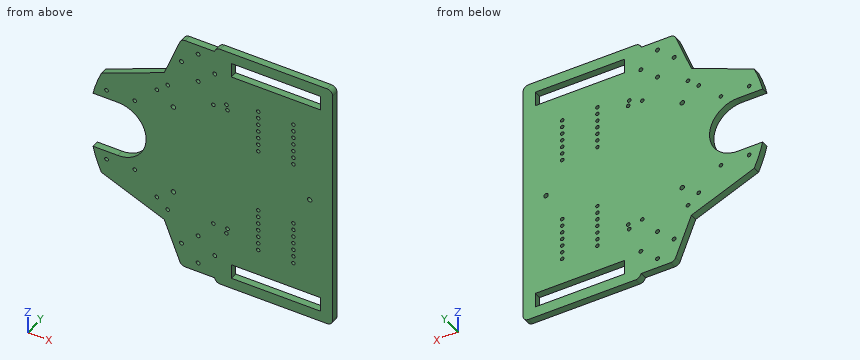
from build123d import *

# Parameters (mm, degrees)
BOSS_EXTRUDE1_DEPTH    = 6.35
SKETCH2_R              = 1.5875
SKETCH2_W              = 80.264
SKETCH2_H              = 12.954
CUT_EXTRUDE1_DEPTH     = 162.484606465
SKETCH7_R              = 2.032
CUT_EXTRUDE4_DEPTH     = 162.484606465
SKETCH8_R              = 1.651
CUT_EXTRUDE5_DEPTH     = 162.484606465
CUT_EXTRUDE6_DEPTH     = 160.416662013
SKETCH10_R             = 1.651
CUT_EXTRUDE7_DEPTH     = 160.416662013
SKETCH11_W             = 225
SKETCH11_H             = 6.35
BOSS_EXTRUDE2_DEPTH    = 8
FILLET2_R              = 5.08
SKETCH15_W             = 29.985408059
SKETCH15_H             = 4.069721463
CUT_EXTRUDE8_DEPTH     = 160.416662013
CUT_EXTRUDE9_START     = -6.35
CUT_EXTRUDE9_OUTLINE_R = 1.775
CUT_EXTRUDE9_DEPTH     = 6.35


# Read off the part's stored shape, not the designer's step: Cut-Extrude9
with BuildPart() as part:
    # Sketch1 → Boss-Extrude1 (new body)
    with BuildSketch(Plane(origin=(0, 0, 0), x_dir=(1, 0, 0), z_dir=(0, 1, 0))):
        with BuildLine():
            Line((-3.175, 112.5), (95.25, 112.5))
            Line((95.25, 112.5), (95.25, -112.5))
            Line((95.25, -112.5), (-3.175, -112.5))
            ThreePointArc((-3.175, -112.5), (-115.675, 0), (-3.175, 112.5))
        make_face()
    extrude(amount=-BOSS_EXTRUDE1_DEPTH)

    # Sketch2 → Cut-Extrude1 (cut, through all)
    with BuildSketch(Plane(origin=(0, 0, 0), x_dir=(1, 0, 0), z_dir=(0, 1, 0))):
        with Locations(Location((36.144045702, -66.3448, 0), (0, 0, 270))):
            Circle(SKETCH2_R)
        with Locations(Location((36.144045702, -59.9948, 0), (0, 0, 270))):
            Circle(SKETCH2_R)
        with Locations(Location((36.144045702, -53.6448, 0), (0, 0, 270))):
            Circle(SKETCH2_R)
        with Locations(Location((36.144045702, -47.2948, 0), (0, 0, 270))):
            Circle(SKETCH2_R)
        with Locations(Location((36.144045702, -40.9448, 0), (0, 0, 270))):
            Circle(SKETCH2_R)
        with Locations(Location((36.144045702, -34.5948, 0), (0, 0, 270))):
            Circle(SKETCH2_R)
        with Locations(Location((36.144045702, -28.2448, 0), (0, 0, 270))):
            Circle(SKETCH2_R)
        with Locations(Location((67.894045702, -66.3448, 0), (0, 0, 270))):
            Circle(SKETCH2_R)
        with Locations(Location((67.894045702, -59.9948, 0), (0, 0, 270))):
            Circle(SKETCH2_R)
        with Locations(Location((67.894045702, -53.6448, 0), (0, 0, 270))):
            Circle(SKETCH2_R)
        with Locations(Location((67.894045702, -47.2948, 0), (0, 0, 270))):
            Circle(SKETCH2_R)
        with Locations(Location((67.894045702, -40.9448, 0), (0, 0, 270))):
            Circle(SKETCH2_R)
        with Locations(Location((67.894045702, -34.5948, 0), (0, 0, 270))):
            Circle(SKETCH2_R)
        with Locations(Location((67.894045702, -28.2448, 0), (0, 0, 270))):
            Circle(SKETCH2_R)
        with Locations(Location((36.144045702, 66.3448, 0), (0, 0, 270))):
            Circle(SKETCH2_R)
        with Locations(Location((36.144045702, 59.9948, 0), (0, 0, 270))):
            Circle(SKETCH2_R)
        with Locations(Location((36.144045702, 53.6448, 0), (0, 0, 270))):
            Circle(SKETCH2_R)
        with Locations(Location((36.144045702, 47.2948, 0), (0, 0, 270))):
            Circle(SKETCH2_R)
        with Locations(Location((36.144045702, 40.9448, 0), (0, 0, 270))):
            Circle(SKETCH2_R)
        with Locations(Location((36.144045702, 34.5948, 0), (0, 0, 270))):
            Circle(SKETCH2_R)
        with Locations(Location((36.144045702, 28.2448, 0), (0, 0, 270))):
            Circle(SKETCH2_R)
        with Locations(Location((67.894045702, 66.3448, 0), (0, 0, 270))):
            Circle(SKETCH2_R)
        with Locations(Location((67.894045702, 59.9948, 0), (0, 0, 270))):
            Circle(SKETCH2_R)
        with Locations(Location((67.894045702, 53.6448, 0), (0, 0, 270))):
            Circle(SKETCH2_R)
        with Locations(Location((67.894045702, 47.2948, 0), (0, 0, 270))):
            Circle(SKETCH2_R)
        with Locations(Location((67.894045702, 40.9448, 0), (0, 0, 270))):
            Circle(SKETCH2_R)
        with Locations(Location((67.894045702, 34.5948, 0), (0, 0, 270))):
            Circle(SKETCH2_R)
        with Locations(Location((67.894045702, 28.2448, 0), (0, 0, 270))):
            Circle(SKETCH2_R)
        with Locations((52.019045702, -96.4438)):
            Rectangle(SKETCH2_W, SKETCH2_H)
        with Locations((52.019045702, 96.4438)):
            Rectangle(SKETCH2_W, SKETCH2_H)
    extrude(amount=-CUT_EXTRUDE1_DEPTH, mode=Mode.SUBTRACT)

    # Sketch7 → Cut-Extrude4 (cut, through all)
    with BuildSketch(Plane(origin=(0, 0, 0), x_dir=(1, 0, 0), z_dir=(0, 1, 0))):
        with Locations(Location((82.511862056, 0, 0), (0, 0, 270))):
            Circle(SKETCH7_R)
        with Locations(Location((-40.297137944, 40.64, 0), (0, 0, 270))):
            Circle(SKETCH7_R)
        with Locations(Location((-40.297137944, -40.64, 0), (0, 0, 270))):
            Circle(SKETCH7_R)
    extrude(amount=-CUT_EXTRUDE4_DEPTH, mode=Mode.SUBTRACT)

    # Sketch8 → Cut-Extrude5 (cut, through all)
    with BuildSketch(Plane(origin=(0, 0, 0), x_dir=(1, 0, 0), z_dir=(0, 1, 0))):
        with Locations(Location((-100.5586, 33.02, 0), (0, 0, 270))):
            Circle(SKETCH8_R)
        with Locations(Location((-100.5586, -33.02, 0), (0, 0, 270))):
            Circle(SKETCH8_R)
        with Locations(Location((-75.1586, 33.02, 0), (0, 0, 270))):
            Circle(SKETCH8_R)
        with Locations(Location((-75.1586, -33.02, 0), (0, 0, 270))):
            Circle(SKETCH8_R)
        with BuildLine():
            Line((-90.2716, 25.4), (-229.776686608, 25.4))
            Line((-229.776686608, 25.4), (-229.776686608, -25.4))
            Line((-229.776686608, -25.4), (-90.2716, -25.4))
            ThreePointArc((-90.2716, -25.4), (-64.8716, 0), (-90.2716, 25.4))
        make_face()
    extrude(amount=-CUT_EXTRUDE5_DEPTH, mode=Mode.SUBTRACT)

    # Sketch9 → Cut-Extrude6 (cut, through all)
    with BuildSketch(Plane(origin=(0, 0, 0), x_dir=(1, 0, 0), z_dir=(0, 1, 0))):
        Polygon((-105.15131959, 47.508738596), (-48.53191541, 70.384462776), (-12.279886537, 160.111382848), (-19.546794421, 160.111382848), (-135.640402248, 160.111382848), (-135.640402248, 47.508738596), align=None)
        Polygon((-105.15131959, -47.508738596), (-48.53191541, -70.384462776), (-12.279886537, -160.111382848), (-135.640402248, -160.111382848), (-135.640402248, -47.508738596), align=None)
    extrude(amount=-CUT_EXTRUDE6_DEPTH, mode=Mode.SUBTRACT)

    # Sketch10 → Cut-Extrude7 (cut, through all)
    with BuildSketch(Plane(origin=(0, 0, 0), x_dir=(1, 0, 0), z_dir=(0, 1, 0))):
        with Locations(Location((-55.150916162, 51.425007473, 0), (0, 0, 270))):
            Circle(SKETCH10_R)
        with Locations(Location((-45.493760399, 59.672997687, 0), (0, 0, 270))):
            Circle(SKETCH10_R)
        with Locations(Location((-4.266941588, 56.871109398, 0), (0, 0, 270))):
            Circle(SKETCH10_R)
        with Locations(Location((7.508293365, 61.628613135, 0), (0, 0, 270))):
            Circle(SKETCH10_R)
        with Locations(Location((8.433058412, -56.871109398, 0), (0, 0, 270))):
            Circle(SKETCH10_R)
        with Locations(Location((8.433058412, 56.871109398, 0), (0, 0, 270))):
            Circle(SKETCH10_R)
        with Locations(Location((-55.150916162, -51.425007473, 0), (0, 0, 270))):
            Circle(SKETCH10_R)
        with Locations(Location((-45.493760399, -59.672997687, 0), (0, 0, 270))):
            Circle(SKETCH10_R)
        with Locations(Location((-4.266941588, -56.871109398, 0), (0, 0, 270))):
            Circle(SKETCH10_R)
        with Locations(Location((7.508293365, -61.628613135, 0), (0, 0, 270))):
            Circle(SKETCH10_R)
    extrude(amount=-CUT_EXTRUDE7_DEPTH, mode=Mode.SUBTRACT)

    # Sketch11 → Boss-Extrude2 (add)
    with BuildSketch(Plane(origin=(95.25, 0, 0), x_dir=(0, 0, -1), z_dir=(1, 0, 0))):
        with Locations((0, -3.175)):
            Rectangle(SKETCH11_W, SKETCH11_H)
    extrude(amount=BOSS_EXTRUDE2_DEPTH)

    # Fillet2
    fillet2_edges = [part.edges().sort_by_distance(p)[0] for p in [
        (103.25, -3.175, -112.5),
        (103.25, -3.175, 112.5),
    ]]
    fillet(fillet2_edges, radius=FILLET2_R)

    # Sketch15 → Cut-Extrude8 (cut, through all)
    with BuildSketch(Plane(origin=(0, 0, 0), x_dir=(1, 0, 0), z_dir=(0, 1, 0))):
        with Locations((-18.16770403, -110.465139268)):
            Rectangle(SKETCH15_W, SKETCH15_H)
        with Locations((-18.16770403, 110.465139268)):
            Rectangle(SKETCH15_W, SKETCH15_H)
    extrude(amount=-CUT_EXTRUDE8_DEPTH, mode=Mode.SUBTRACT)

    # Cut-Extrude9 outline → Cut-Extrude9 (cut)
    with BuildSketch(Plane(origin=(0, 0, 0), x_dir=(1, 0, 0), z_dir=(0, 1, 0)).offset(CUT_EXTRUDE9_START)):
        with BuildLine():
            Line((-3.175, 112.5), (-3.175, 108.430278537))
            ThreePointArc((-3.175, 108.430278537), (-1.411607293, 111.353104052), (1.803527622, 112.5))
            Line((1.803527622, 112.5), (-3.175, 112.5))
        make_face()
        with BuildLine():
            ThreePointArc((-34.443998775, 105.253280031), (-32.574604743, 107.561789405), (-29.733904794, 108.430278537))
            Line((-29.733904794, 108.430278537), (-33.160408059, 108.430278537))
            Line((-33.160408059, 108.430278537), (-34.443998775, 105.253280031))
        make_face()
        with BuildLine():
            Line((-33.160408059, -108.430278537), (-29.733904794, -108.430278537))
            ThreePointArc((-29.733904794, -108.430278537), (-32.574604743, -107.561789405), (-34.443998775, -105.253280031))
            Line((-34.443998775, -105.253280031), (-33.160408059, -108.430278537))
        make_face()
        with BuildLine():
            ThreePointArc((1.803527622, -112.5), (-1.411607293, -111.353104052), (-3.175, -108.430278537))
            Line((-3.175, -108.430278537), (-3.175, -112.5))
            Line((-3.175, -112.5), (1.803527622, -112.5))
        make_face()
        with Locations((-33, -87)):
            Circle(CUT_EXTRUDE9_OUTLINE_R)
        with Locations((-18, -100)):
            Circle(CUT_EXTRUDE9_OUTLINE_R)
        with Locations((-18, -74)):
            Circle(CUT_EXTRUDE9_OUTLINE_R)
        with Locations((-3, -87)):
            Circle(CUT_EXTRUDE9_OUTLINE_R)
        with Locations((-33, 87)):
            Circle(CUT_EXTRUDE9_OUTLINE_R)
        with Locations((-18, 100)):
            Circle(CUT_EXTRUDE9_OUTLINE_R)
        with Locations((-18, 74)):
            Circle(CUT_EXTRUDE9_OUTLINE_R)
        with Locations((-3, 87)):
            Circle(CUT_EXTRUDE9_OUTLINE_R)
    extrude(amount=CUT_EXTRUDE9_DEPTH, mode=Mode.SUBTRACT)


solid = part.part
Could you check a few things on this model? Use its own coordinates, in mm. Give positions to 0.01 mm unless a question says otherwise; leave off trailing zeros. Order: outer loops, then holes, each group sorted by start corner. A loop starts at its lowest first (then second) coordinate and runs counter-clockwise, first axis right, second up. Notation, with made-up numbers: (-39.75, -10) -> (7.25, -10) arc R19 ccw to (7.25, 6) -> close; hole circle Ø2 at (0, 73). An arc over 180 degrees is marked (long way). Answer in a Markdown table with one row per item. Add a question column.
Item 1: Please list where these lines run through material, in increasing order: probe 1 along Z at (x, y) = (88, -0.5); probe 2 along Z at (x, y) = (-74.5, -4); probe 3 along Z at (x, y) = (-54, -2).
Item 2: Imagine slicing it at C-C (y = -4.5). Count the separate pieces of the cut face and the enclosed holes in it, and give its area (3 significant figures).
Item 3: Imagine slicing it at A-A (x = 57). List the corners of the cut face in (y, z) for me, and give its area (3 significant figures).
Item 4: Imagine slicing it at D-D (z = -82). List the corners of the cut face in (x, y) for me.
Item 5: I'm going to push flat-ended pins straight in: P1, Ø5.5, axis at x = 7.51, z = 61.63, coming from the -Y side; P2, Ø1.9, axis at x = -98.5, y = -2, coming from the -Z side; P3, Ø2.5, axis at x = 67.89, z = -59.99, coming from the -Y side; P4, Ø1.9, axis at y = -2, z = -98, coming from the -X side. Where does each tip first touch, or does it pass through?
Item 6: Imagine slicing it at B-B (x = -80.5). List the corners of the cut face in (y, z) for me.
Result:
| question | item | result |
|---|---|---|
| 1 | probe 1 | -112.5 to -102.92, -89.97 to 89.97, 102.92 to 112.5 |
| 1 | probe 2 | -59.89 to -34.53, -31.51 to -19.91, 19.91 to 31.51, 34.53 to 59.89 |
| 1 | probe 3 | -68.18 to -52.61, -50.24 to 50.24, 52.61 to 68.18 |
| 2 | separate pieces | 1 |
| 2 | enclosed holes | 55 |
| 2 | area | 35,700 mm2 |
| 3 | outline | (-6.35, -112.5) -> (0, -112.5) -> (0, -102.92) -> (-6.35, -102.92) -> close; (-6.35, -89.97) -> (0, -89.97) -> (0, 89.97) -> (-6.35, 89.97) -> close; (-6.35, 102.92) -> (0, 102.92) -> (0, 112.5) -> (-6.35, 112.5) -> close |
| 3 | area | 1,260 mm2 |
| 4 | outline | (-43.84, -6.35) -> (103.25, -6.35) -> (103.25, 0) -> (-43.84, 0) -> close |
| 5 | P1 | y = -6.35 |
| 5 | P2 | z = -50.58 |
| 5 | P3 | through |
| 5 | P4 | x = -37.76 |
| 6 | outline | (-6.35, -57.47) -> (0, -57.47) -> (0, -23.45) -> (-6.35, -23.45) -> close; (-6.35, 23.45) -> (0, 23.45) -> (0, 57.47) -> (-6.35, 57.47) -> close |
